Verification items for the finished model (mm, model axes). Coordinates: 2 decimals unless noted, no trailing zeros. Write each loop counter-clockwise with the first axis right and the second up, starting at its lowest first coordinate (ties: lowest second). Pieces come first, ordered by that corner, then holes.
```python
from build123d import *

# Parameters (mm, degrees)
F0_R     = 20
F1_DEPTH = 3
F2_R     = 20.25
F2_R_2   = 20
F3_DEPTH = 3
F5_DEPTH = 0.2
F6_R     = 1.5
F7_R     = 11
F7_R_2   = 8
F8_DEPTH = 20


with BuildPart() as f1:
    # F0 (on Top) → F1 (new body)
    with BuildSketch(Plane.XY):
        Circle(F0_R)
    extrude(amount=F1_DEPTH)

    # F2 (on face) → F3 (cut)
    with BuildSketch(Plane(origin=(0, 0, 0), x_dir=(1, 0, 0), z_dir=(0, 0, -1))):
        Circle(F2_R)
        Circle(F2_R_2, mode=Mode.SUBTRACT)
    extrude(amount=-F3_DEPTH, mode=Mode.SUBTRACT)

    # F4 (on face) → F5 (cut)
    with BuildSketch(Plane.XY.offset(3)):
        Polygon((-6.553545, 6.441406), (-10.126568, 4.57168), (-8.068945, 11.901424), (-15.633037, 4.746201), (-13.924567, -5.449917), (-2.965713, -0.560796), (-5.021182, 2.150405), (-11.850991, -2.621582), (-13.342778, 0.3595), (-10.126568, 0.808129), align=None)
        Polygon((-2.489465, 14.390621), (4.339508, 11.025493), (0.561338, 9.6156), (7.140174, 8.511416), (9.622473, 10.605087), (10.844337, 7.503583), (2.730879, 5.608866), (3.375366, 2.268177), (14.33422, 7.157298), (7.887996, 15.239742), align=None)
        Polygon((-0.990919, 3.307807), (-3.394604, 3.307807), (-2.691304, -0.438372), (3.029758, 2.113989), (0.458553, 4.941968), align=None)
        Polygon((1.963912, -7.359985), (2.05385, -7.474527), (3.964488, -7.474527), (5.622064, -6.417363), (5.452343, -5.734665), (8.692019, -5.561052), (8.814289, -4.11721), (8.372472, -4.618176), (5.173013, -4.720715), (4.874605, -3.637509), (8.333541, -3.403418), (8.333541, -1.885541), (7.824205, -2.463065), (4.551061, -2.463065), (4.272204, -1.450831), (7.780703, -1.253439), (7.887996, 0.240209), (7.347112, -0.279066), (3.964488, -0.333842), (3.693176, 0.651006), (7.265975, 0.808129), (7.54025, 2.389176), (7.140174, 1.96216), (3.320525, 1.903422), (-2.747671, -0.803809), (-4.885467, -3.637509), (-5.783685, -3.637509), (-4.438388, -4.488719), (-2.104728, -2.178321), (-1.484141, -2.968676), (-3.652246, -5.282777), (-4.438388, -5.294866), (-3.170688, -6.251243), (-0.771632, -3.876101), (-0.136667, -4.684767), (-2.260593, -6.990367), (-3.052734, -6.990367), (-1.825474, -7.983332), (0.561338, -5.57372), (1.270919, -6.477416), (-0.771632, -8.778695), (-1.6229, -8.778695), (-0.392072, -9.644426), align=None)
        Polygon((3.985386, -7.864483), (2.199684, -7.864483), (2.073994, -11.069699), (3.102296, -11.682914), (5.501691, -11.554331), (5.622064, -6.820647), align=None)
        Polygon((3.029758, -12.026839), (1.876301, -11.338989), (-0.136667, -13.621443), (0.230974, -14.74811), (1.653607, -15.934166), (5.380382, -11.90087), align=None)
        Polygon((-0.101783, -15.026066), (-0.392072, -13.858383), (-3.294068, -14.80533), (-3.612137, -15.766781), (-3.170688, -16.971571), (1.190486, -16.220126), align=None)
        Polygon((-7.284677, -12.611533), (-8.39267, -13.017515), (-3.574296, -17.034617), (-4.038847, -15.766781), (-3.701848, -14.74811), align=None)
        Polygon((-10.419287, -13.290767), (-7.436289, -12.19776), (-8.068945, -6.186221), align=None)
    extrude(amount=-F5_DEPTH, mode=Mode.SUBTRACT)

    # F6
    f6_edges = [f1.edges().sort_by_distance(p)[0] for p in [
        (-20, 0, 3),
    ]]
    fillet(f6_edges, radius=F6_R)

    # F7 (on face) → F8 (join)
    with BuildSketch(Plane(origin=(0, 0, 0), x_dir=(1, 0, 0), z_dir=(0, 0, -1))):
        Circle(F7_R)
        Circle(F7_R_2, mode=Mode.SUBTRACT)
    extrude(amount=F8_DEPTH)


solid = f1.part
```
1. Material ranges on L1, parallel to X at y = 0, z = -10.75; L2, parallel to Z at x = 11.5, y = 0, recorded low to high.
2. Sectioned sample at A-A, the plane z = -13.5. Record the boundary of the cut face in (x, y).
3. Draft check along Y on faces 1 (the flat face through (0, 2, 2.8)), 2 (the flat face through (-2, 8, -20)), 3 (the cylindrical face through (-4.336, -19.524, 0.74)). Enter one of: pulls with the +Y half, pulls with the -Y half, needs draft (parallel to the pull), parting line crosses it, or undercut.
4. Gauge pin test, flat ends, axial feed: P1, Ø5, axis at x = 14.5, y = 8, coming from the -Z side; P2, Ø4, axis at x = -0.5, z = -14, coming from the -Y side; P3, Ø5, axis at y = 12, z = -13, coming from the +X side. Record the tip position at first contact, or that the pin passes through.
Outcome:
1. L1: x = -11 to -8, 8 to 11
1. L2: z = 0 to 3
2. outline: circle Ø22 at (0, 0); hole circle Ø16 at (0, 0)
3. face 1: undercut
3. face 2: needs draft
3. face 3: parting line crosses it
4. P1: stops at z = 0
4. P2: stops at y = -11
4. P3: stops at x = 5.55
